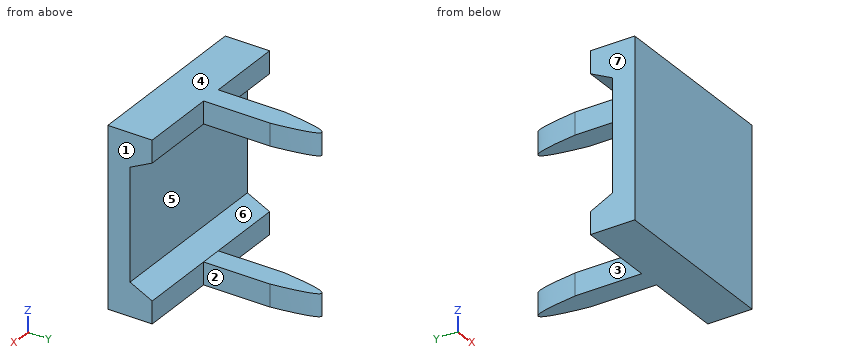
```python
from build123d import *

# Parameters (mm, degrees)
SKETCH2_W               = 80
SKETCH2_H               = 80
BOSS_EXTRUDE1_DEPTH     = 20
BOSS_EXTRUDE2_DEPTH     = 10
CUT_EXTRUDE1_DEPTH      = 134.041347129
CUT_EXTRUDE1_DEPTH_BACK = 134.041347129


with BuildPart() as part:
    # Sketch2 → Boss-Extrude1 (new body)
    with BuildSketch(Plane(origin=(0, 0, 0), x_dir=(1, 0, 0), z_dir=(0, 1, 0))):
        with Locations((40, 40)):
            Rectangle(SKETCH2_W, SKETCH2_H)
    extrude(amount=BOSS_EXTRUDE1_DEPTH)

    # Sketch3 → Boss-Extrude2 (add)
    with BuildSketch(Plane.XY):
        with BuildLine():
            Line((35, 20), (35, 50))
            add(Edge.make_bspline(
                [(35, 50), (40, 90), (45, 50)],
                knots=[0, 0, 0, 1, 1, 1], degree=2))
            Line((45, 50), (45, 20))
            Line((45, 20), (35, 20))
        make_face()
    boss_extrude2 = extrude(amount=-BOSS_EXTRUDE2_DEPTH)

    # Mirror1: Boss-Extrude2 across plane
    add(boss_extrude2.mirror(Plane.XY.offset(-40)))

    # Sketch4 → Cut-Extrude1 (cut, two sides: drawn at the far end of the back side and taken through both)
    with BuildSketch(Plane(origin=(80, 0, 0), x_dir=(0, 0, -1), z_dir=(1, 0, 0)).offset(-CUT_EXTRUDE1_DEPTH_BACK)):
        Polygon((70, 20), (10, 20), (15, 10), (65, 10), align=None)
    extrude(amount=CUT_EXTRUDE1_DEPTH + CUT_EXTRUDE1_DEPTH_BACK, mode=Mode.SUBTRACT)


solid = part.part
```
Could you check a few things on this model? Use its own coordinates, in mm. Face numbers are marked on the shaded views. A direction names the side the tool comes from. Round coordinates to 2 decimals unless told otherwise and drop trailing zeros. Loops run counter-clockwise (first coordinate to the right, second up) from the corner with the lowest first, then second, coordinate; pieces in that order, holes last. Notation, with made-up numbers: (84.5, -21.75) - (143.5, -21.75) arc R29 ccw to (143.5, 8.25) - close; hole circle Ø6 at (49.25, -13). An arc over 180 degrees is marked (long way). Answer as CSV lines item,"result".
1. On a 3-axis mill with a long thin cutter (end or side, diameter ignored), from which of +Z, -Z, +X, -X, +Y, -Y can I reach the whole of each face in a straight line? I mean the marked faces 1, 2 and 3. Say none if no direction works.
Filled in:
face 1,"+Z, -Z, +X, +Y, -Y"
face 2,"+Z, -Z, +X, +Y"
face 3,"+Z, -Z, -X, +Y"
2. I want a section at A-A on y = 36.5. List the corners of the cut face in (x, z) for me.
Filled in:
outline,"(35, -80) - (45, -80) - (45, -70) - (35, -70) - close; (35, -10) - (45, -10) - (45, 0) - (35, 0) - close"
3. For pin 1 Ø8 at (x, z) = (12, -6) entering from +Y; pin 2 Ø5 at (y, z) = (32.5, -5) entering from -X; pin 3 Ø11 at (y, z) = (38, -7) entering from +X, each with a flat end and sliding along its axis, tell me the tip position at first contact or that it passes through.
Filled in:
pin 1,"stops at y = 20"
pin 2,"stops at x = 35"
pin 3,"stops at x = 45"
4. I want a section at C-C on z = -48.5. List the corners of the cut face in (x, y) for me.
Filled in:
outline,"(0, 0) - (80, 0) - (80, 10) - (0, 10) - close"
5. I want a section at B-B on x = 59.5. List the corners of the cut face in (y, z) for me.
Filled in:
outline,"(0, -80) - (20, -80) - (20, -70) - (10, -65) - (10, -15) - (20, -10) - (20, 0) - (0, 0) - close"
6. We'd pull the mould along Z, two halves only. Please class the marked faces 4, 5, 6 and 7: +Z half, -Z half, draft (parallel to the pull), parting line (faces both ways), or undercut.
Filled in:
face 4,"+Z half"
face 5,"undercut"
face 6,"undercut"
face 7,"draft"
7. Please list where these lines run through material, in increasing order: line 1 along Y through (x, z) = (29, -60); line 2 along Y through (x, z) = (5, -73); line 3 along X through (y, z) = (48, -72.5). Write a range as [from, to].
Filled in:
line 1,"y = [0, 10]"
line 2,"y = [0, 20]"
line 3,"x = [35, 45]"
